Part print with two shaded views. Sizes in mm from the minimum x, y, z corner. Coordinates: 2 decimals unless noted, no trailing zeros. Write each loop counter-clockwise with the first axis right and the second up, starting at its lowest first coordinate (ties: lowest second). Pieces come first, ordered by that corner, then holes. Notation, with made-up numbers: (38, 6) - (93, 6) arc R14 cw to (93, 13) - close; hole circle Ø3 at (38.5, -1.5). An arc over 180 degrees is marked (long way). Answer in a Markdown table with one row per item. Add a question column.
Q1. Pin check, flat tip, straight feed: pin 1 (1.8 mm diameter, centred on x = 34.5, y = 38, fed in from +Z). Stop position of the tip, or through.
Q2. Drill centre lines: line 1 along X through (y, z) = (71.5, 3.9); line 2 along Z through (x, y) = (37, 25.5); line 3 along Y through (x, z) = (48.5, 4.85). Where is each one in solid material? Low to high. Write a range as from..to.
Q3. Band-saw the part on A-A (y = 46). List the corners of the cut face in (x, z), and give its area (3 significant figures).
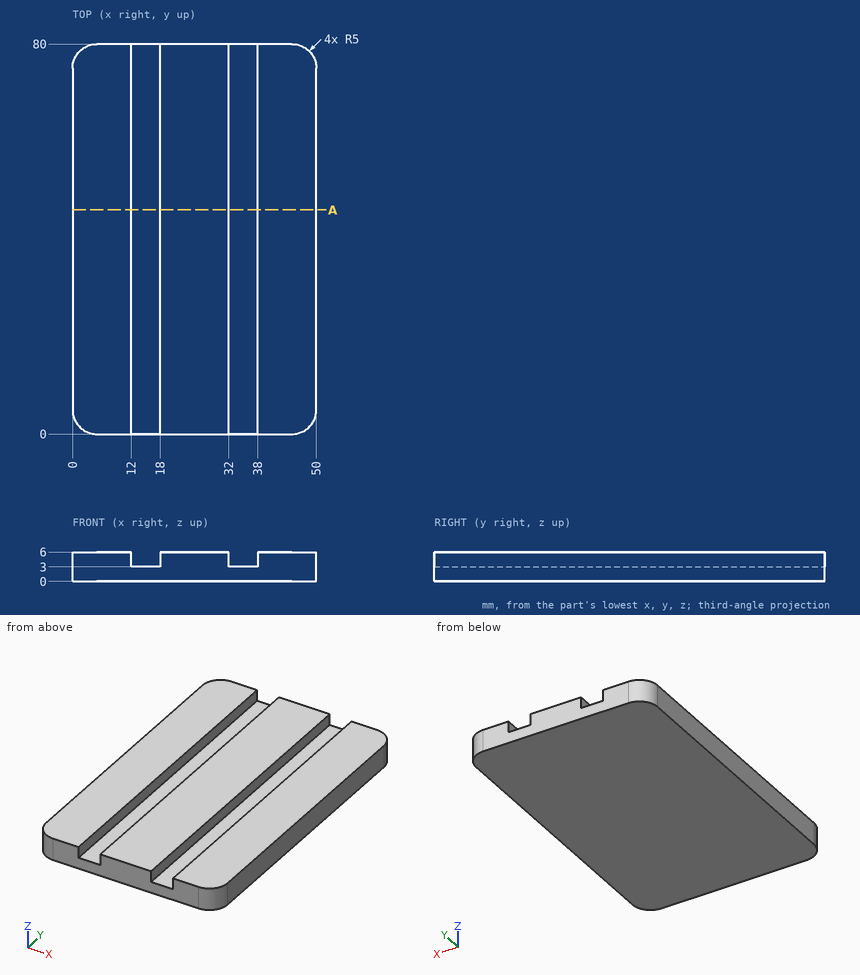
Checked values:
| question | item | result |
|---|---|---|
| 1 | pin 1 | stops at z = 3 |
| 2 | line 1 | x = 0..12, 18..32, 38..50 |
| 2 | line 2 | z = 0..3 |
| 2 | line 3 | y = 1.43..78.57 |
| 3 | outline | (0, 0) - (50, 0) - (50, 6) - (38, 6) - (38, 3) - (32, 3) - (32, 6) - (18, 6) - (18, 3) - (12, 3) - (12, 6) - (0, 6) - close |
| 3 | area | 264 mm² |
